Read the model definition and answer for the solid it produces. Units are mm, in the model's axes. Coordinates: 2 decimals unless noted, no trailing zeros. Write each loop counter-clockwise with the first axis right and the second up, starting at its lowest first coordinate (ties: lowest second). Pieces come first, ordered by that corner, then holes. Notation, with made-up numbers: (55.5, 33.25) -> (66.5, 33.25) arc R18 ccw to (66.5, 43.25) -> close; hole circle Ø10 at (32.25, 5). An arc over 180 degrees is marked (long way). Use CSV: the item, a comma, the result in double quotes. Start each with the question number.
from build123d import *

# Parameters (mm, degrees)
F0_W     = 101.6
F0_H     = 203.2
F1_DEPTH = 19.05
F3_DEPTH = 19.051
F4_R     = 19.05
F5_DEPTH = 19.051


# Not quite as in the source:
# - a feature names something its author has since deleted; it is built from what else it names


with BuildPart() as f1:
    # F0 (on Front) → F1 (new body)
    with BuildSketch(Plane.XZ):
        Rectangle(F0_W, F0_H)
    extrude(amount=F1_DEPTH)

    # F2 (on face) → F3 (cut, through all)
    with BuildSketch(Plane.XZ.offset(19.05)):
        Polygon((-50.8, 44.8038733715), (0, 101.6), (-50.8, 101.6), align=None)
        Polygon((50.8, 101.6), (0, 101.6), (50.8, 44.8038733715), align=None)
    extrude(amount=-F3_DEPTH, mode=Mode.SUBTRACT)

    # F4 (on face) → F5 (cut, through all)
    with BuildSketch(Plane.XZ.offset(19.05)):
        Circle(F4_R)
    extrude(amount=-F5_DEPTH, mode=Mode.SUBTRACT)


solid = f1.part
1) This flat-tipped pin is pushed along its axis until it touches: pin 1 (10 mm diameter, centred on x = -37, y = -12, fed in from +Z). Where does it stop, or does it pass through?
2) Section D-D, the plane z = 85 is taken. Give the vertices of the cut face in (x, y), plus the area to 3 significant figures.
3) Section A-A, the plane z = 0 is taken. Give the vertices of the cut face in (x, y).
4) Find the intervals of material crossed by line 1 along Z through (x, y) = (0, -4.5); line 2 along Z through (x, y) = (-8, -7.25); line 3 along X through (y, z) = (-3, 17.5), in increasing order.
5) Section C-C, the plane y = -9 is taken. Give the vertices of the cut face in (x, z).
6) Section B-B, the plane x = 5 is taken. Give the vertices of the cut face in (y, z).
7) The mould has two halves that part along Z. Classify faces 1 (the face through (-1, -9, -101.6)), 2 (the face through (-15.12, -9.66, -11.59)), 3 (the face through (-1, -19.05, -21)): pulls with the +Z half, pulls with the -Z half, needs draft (parallel to the pull), parting line crosses it, or undercut.
The answers:
1,pin 1,"stops at z = 65.82"
2,outline,"(-14.85, -19.05) -> (14.85, -19.05) -> (14.85, 0) -> (-14.85, 0) -> close"
2,area,"566 mm^2"
3,outline,"(-50.8, -19.05) -> (-19.05, -19.05) -> (-19.05, 0) -> (-50.8, 0) -> close; (19.05, -19.05) -> (50.8, -19.05) -> (50.8, 0) -> (19.05, 0) -> close"
4,line 1,"z = -101.6 to -19.05, 19.05 to 101.6"
4,line 2,"z = -101.6 to -17.29, 17.29 to 92.66"
4,line 3,"x = -50.8 to -7.53, 7.53 to 50.8"
5,outline,"(-50.8, -101.6) -> (50.8, -101.6) -> (50.8, 44.8) -> (0, 101.6) -> (-50.8, 44.8) -> close; hole circle Ø38.1 at (0, 0)"
6,outline,"(-19.05, -101.6) -> (0, -101.6) -> (0, -18.38) -> (-19.05, -18.38) -> close; (-19.05, 18.38) -> (0, 18.38) -> (0, 96.01) -> (-19.05, 96.01) -> close"
7,face 1,"pulls with the -Z half"
7,face 2,"undercut"
7,face 3,"needs draft"
